```python
from build123d import *

# Parameters (mm, degrees)
SKETCH3_R               = 1.25
CUT_EXTRUDE1_DEPTH      = 9
CUT_EXTRUDE2_DEPTH      = 1
CUT_EXTRUDE3_DEPTH      = 15
CUT_EXTRUDE3_DEPTH_BACK = 1
CUT_EXTRUDE3_START      = -40
SKETCH5_W               = 42.611665196
SKETCH5_H               = 2.5


with BuildPart() as part:
    # Sketch2 → Revolve1 (revolve)
    with BuildSketch(Plane(origin=(0, 0, 0), x_dir=(0, 0, -1), z_dir=(1, 0, 0))):
        Polygon((-16, 12), (-16, 9), (-6.75, 9), (-6.75, -9), (-16, -9), (-16, -12), (-6.5, -12), (-6.5, -14), (-4.5, -14), (-4.5, -12), (-4.5, 12), align=None)
    revolve(axis=Axis((0, 15.5, 0), (0, -1, 0)))

    # Sketch3 → Cut-Extrude1 (cut)
    with BuildSketch(Plane.XZ.offset(12)):
        with Locations(Location((0, 8, 0), (0, 0, 270))):
            Circle(SKETCH3_R)
        with Locations(Location((7.425425002, 10.973858189, 0), (0, 0, 270))):
            Circle(SKETCH3_R)
    extrude(amount=-CUT_EXTRUDE1_DEPTH, mode=Mode.SUBTRACT)

    # Sketch4 → Cut-Extrude2 (cut)
    with BuildSketch(Plane(origin=(0, 12, 0), x_dir=(1, 0, 0), z_dir=(0, 1, 0))):
        Polygon((-2.25827734, 10.75), (1.74172266, 10.75), (1.74172266, 13.000000233), (4.74172266, 10), (1.74172266, 7.000000233), (1.74172266, 9.25), (-2.25827734, 9.25), align=None)
    extrude(amount=-CUT_EXTRUDE2_DEPTH, mode=Mode.SUBTRACT)

    # Sketch5 → Cut-Extrude3 (cut, two sides: drawn at the far end of the back side and taken through both)
    with BuildSketch(Plane.XZ.offset(14).offset(CUT_EXTRUDE3_START - CUT_EXTRUDE3_DEPTH_BACK)):
        Rectangle(SKETCH5_W, SKETCH5_H)
    extrude(amount=CUT_EXTRUDE3_DEPTH + CUT_EXTRUDE3_DEPTH_BACK, mode=Mode.SUBTRACT)


solid = part.part
```
Design review of the part built by this model. Coordinates are the model's own, in mm. A direction names the side the tool comes from. Coordinates: 2 decimals unless noted, no trailing zeros. Loops run counter-clockwise (first coordinate to the right, second up) from the corner with the lowest first, then second, coordinate; pieces in that order, holes last. Notation, with made-up numbers: M -1,54.25 L 22,54.25 A6 ccw 22,59.25 Z; hole C 39,-7 d1. An arc over 180 degrees is marked long. One line per question, with ' | ' between items.
(1) Wall thickness on probe 1 along Y at (x, z) = (-6, 12.5); probe 2 along Z at (x, y) = (0, 4): over which ranges is each line inside the solid? List them lowest first.
Filled in:
probe 1: y = -12 to -9, 9 to 12 | probe 2: z = -6.75 to -4.5, 4.5 to 6.75
(2) Machinability: for faces 1 (the face through (15.62, -10.52, -3.47)), 2 (the face through (7, -12, 0)), 3 (the face through (-0.2, 11.5, -9.25)), 4 (the face through (10.1, 11.5, 1.25)), which of the approach directions +Z, -Z, +X, -X, +Y, -Y give a long, thin tool a straight path to every point of the face, cutting with its end or side? Answer none if there is none.
Filled in:
face 1: +Y, -Y | face 2: -Y | face 3: +Y | face 4: +X, -X, +Y
(3) For pin 1 Ø0.5 at (x, y) = (-1, 11.5) entering from +Z; pin 2 Ø10 at (x, y) = (-11.5, 9.5) entering from +Z; pin 3 Ø1.5 at (y, z) = (4, 1.5) entering from -X; pin 4 Ø8 at (x, z) = (0, 0) entering from -Y, all flat-tipped, find the tip position at first contact; note any pin that passes through.
Filled in:
pin 1: stops at z = 15.98 | pin 2: stops at z = 14.62 | pin 3: stops at x = -6.71 | pin 4: passes through
(4) We need section D-D (y = 2). Give the boundary of the cut face in (x, z).
Filled in:
outline: C 0,0 d13.5; hole C 0,0 d9
(5) Draft analysis for pull direction Z (two halves, no side actions). For faces 5 (the face through (6.59, -0.13, -1.46)), 6 (the face through (0, -9, -7)), 7 (the face through (-10.2, 11.5, 1.25)), state which applies: released by +Z, released by -Z, zero draft, split by the parting line, or undercut.
Filled in:
face 5: split by the parting line | face 6: zero draft | face 7: undercut
(6) We need section B-B (x = -11). Give the boundary of the cut face in (y, z).
Filled in:
outline: M -12,-11.62 L -9,-11.62 L -9,11.62 L -12,11.62 Z; M 9,-11.62 L 12,-11.62 L 12,-1.25 L 11,-1.25 L 11,1.25 L 12,1.25 L 12,11.62 L 9,11.62 Z
(7) We need section A-A (z = 0). Give the boundary of the cut face in (x, y).
Filled in:
outline: M -16,-12 L -6.5,-12 L -6.5,-14 L -4.5,-14 L -4.5,11 L -16,11 L -16,9 L -6.75,9 L -6.75,-9 L -16,-9 Z; M 4.5,-14 L 6.5,-14 L 6.5,-12 L 16,-12 L 16,-9 L 6.75,-9 L 6.75,9 L 16,9 L 16,11 L 4.5,11 Z
(8) We need section C-C (z = 8). Give the boundary of the cut face in (x, y).
Filled in:
outline: M -13.86,-12 L -1.25,-12 L -1.25,-9 L -13.86,-9 Z; M -13.86,9 L 13.86,9 L 13.86,12 L -13.86,12 Z; M 1.25,-12 L 13.86,-12 L 13.86,-9 L 1.25,-9 Z
